Can you work these out from the model? Positions are in its coordinate system, mm. Face numbers are marked on the shaded views. Give positions to 0.01 mm unless a question says otherwise; leave off trailing zeros. Write each loop counter-clockwise with the first axis right and the second up, starting at its lowest first coordinate (ties: lowest second). Pieces come first, ordered by that corner, then holes. Notation, with made-up numbers: (20.25, 33) -> (42.25, 33) arc R30 ccw to (42.25, 61) -> close; hole circle Ø2 at (70, -38). An arc over 180 degrees is marked (long way). Answer as CSV lines item,"result". Start each with the question number.
1. If we mould it in two halves opening along X, with no side actions, what happens to the marked faces 1 and 2? For each: pulls with the +X half, pulls with the -X half, needs draft (parallel to the pull), parting line crosses it, or undercut.
2. I need wall thicknesses on line 1 (Z direction, x = 0, y = 8.3); line 2 (Y direction, x = -11.5, z = 0.5). Which ranges of each line are inside material? Lowest first, please. Write a range as [from, to].
3. If we section it at D-D on z = -14.5: Write out the boundary of the cut face in (x, y), plus the area to 3 significant figures.
4. If we section it at C-C on y = 4.75: Write out the boundary of the cut face in (x, z), plus the area to 3 significant figures.
5. If we section it at B-B on x = 0: Write out the boundary of the cut face in (y, z), plus the area to 4 significant figures.
6. If we section it at A-A on z = 0: Write out the boundary of the cut face in (x, y).
7. I'm going to push flat-ended pins straight in: P1, Ø12.5, axis at x = 0, z = 0, coming from the +Y side; P2, Ø3, axis at y = 8, z = -6, coming from the +X side; P3, Ø0.6, axis at x = 17, z = -9.5, coming from the -Y side; P4, Ø2, axis at y = 1.5, z = 1.5, coming from the -X side. Where does each tip first touch, or does it pass through?
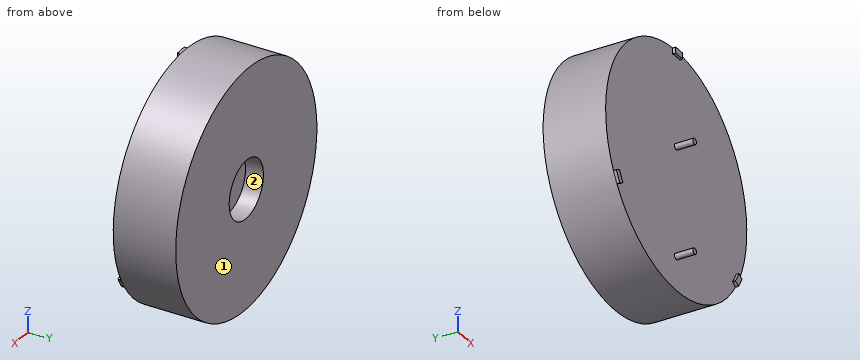
```python
from build123d import *
from build123d.topology import SkipClean

# Parameters (mm, degrees)
BOSS_EXTRUDE1_START = 0.5
BOSS_EXTRUDE1_DEPTH = 0.5
SKETCH3_R           = 0.5
BOSS_EXTRUDE2_DEPTH = 3.1


with BuildPart() as part:
    # Sketch1 → Revolve1 (revolve)
    with BuildSketch(Plane(origin=(0, 0, 0), x_dir=(0, 0, -1), z_dir=(1, 0, 0))):
        Polygon((20.2, 10.5), (20.2, 0), (0, 0), (0, 7.5), (4.9, 7.5), (4.9, 10.5), align=None)
    revolve(axis=Axis((0, 0, 0), (0, 1, 0)))

    # Sketch2 → Boss-Extrude1 (add)
    with SkipClean():  # the faces are left unmerged after this step: merging them gives an invalid solid
        with BuildSketch(Plane.XZ.offset(BOSS_EXTRUDE1_START)):
            with BuildLine():
                Line((-1, 20.175232341), (-1, 19.173940649))
                ThreePointArc((-1, 19.173940649), (0, 19.2), (1, 19.173940649))
                Line((1, 19.173940649), (1, 20.175232341))
                ThreePointArc((1, 20.175232341), (0, 20.2), (-1, 20.175232341))
            make_face()
            with BuildLine():
                Line((17.972263734, -9.221590767), (17.105119692, -8.720944921))
                ThreePointArc((17.105119692, -8.720944921), (16.627687753, -9.6), (16.105119692, -10.452995728))
                Line((16.105119692, -10.452995728), (16.972263734, -10.953641574))
                ThreePointArc((16.972263734, -10.953641574), (17.493713156, -10.1), (17.972263734, -9.221590767))
            make_face()
            with BuildLine():
                Line((-16.972263734, -10.953641574), (-16.105119692, -10.452995728))
                ThreePointArc((-16.105119692, -10.452995728), (-16.627687753, -9.6), (-17.105119692, -8.720944921))
                Line((-17.105119692, -8.720944921), (-17.972263734, -9.221590767))
                ThreePointArc((-17.972263734, -9.221590767), (-17.493713156, -10.1), (-16.972263734, -10.953641574))
            make_face()
        extrude(amount=-BOSS_EXTRUDE1_DEPTH)

    # Sketch3 → Boss-Extrude2 (add)
    with SkipClean():  # the faces are left unmerged after this step: merging them gives an invalid solid
        with BuildSketch(Plane.XZ):
            with Locations(Location((0, 4, 0), (0, 0, 270))):
                Circle(SKETCH3_R)
            with Locations(Location((0, -14.5, 0), (0, 0, 270))):
                Circle(SKETCH3_R)
        extrude(amount=BOSS_EXTRUDE2_DEPTH)


solid = part.part
```
Computed values:
1,face 1,"needs draft"
1,face 2,"undercut"
2,line 1,"z = [-20.2, -4.9], [4.9, 20.2]"
2,line 2,"y = [0, 10.5]"
3,outline,"(-14.06, 0) -> (-0.5, 0) -> (-0.5, -3.1) -> (0.5, -3.1) -> (0.5, 0) -> (14.06, 0) -> (14.06, 10.5) -> (-14.06, 10.5) -> close"
3,area,"298 mm2"
4,outline,"circle Ø40.4 at (0, 0)"
4,area,"1,280 mm2"
5,outline,"(-3.1, -15) -> (0, -15) -> (0, -20.2) -> (10.5, -20.2) -> (10.5, -4.9) -> (7.5, -4.9) -> (7.5, 4.9) -> (10.5, 4.9) -> (10.5, 20.2) -> (-0.5, 20.2) -> (-0.5, 19.2) -> (0, 19.2) -> (0, 4.5) -> (-3.1, 4.5) -> (-3.1, 3.5) -> (0, 3.5) -> (0, -14) -> (-3.1, -14) -> close"
5,area,"401.5 mm2"
6,outline,"(-20.2, 0) -> (20.2, 0) -> (20.2, 10.5) -> (4.9, 10.5) -> (4.9, 7.5) -> (-4.9, 7.5) -> (-4.9, 10.5) -> (-20.2, 10.5) -> close"
7,P1,"stops at y = 10.5"
7,P2,"stops at x = 19.69"
7,P3,"stops at y = -0.5"
7,P4,"stops at x = -20.19"
